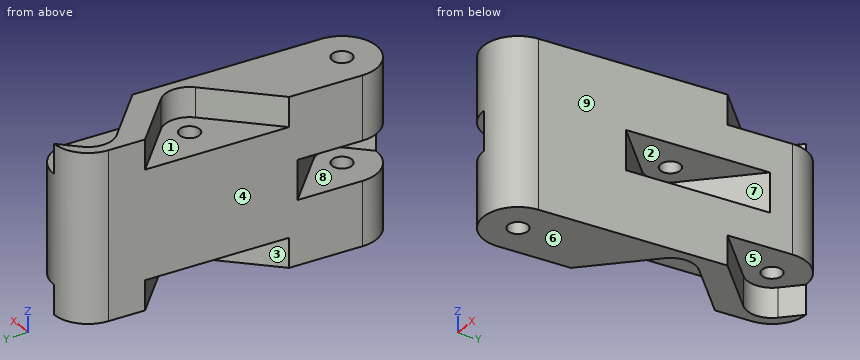
from build123d import *

# Parameters (mm, degrees)
SKETCH1_R           = 1
BOSS_EXTRUDE1_DEPTH = 8.5
CUT_EXTRUDE1_DEPTH  = 2
CUT_EXTRUDE2_START  = -3
CUT_EXTRUDE2_DEPTH  = 3


with BuildPart() as part:
    # Sketch1 → Boss-Extrude1 (new body)
    with BuildSketch(Plane.XY):
        with BuildLine():
            Line((12.42679356, 42.170979879), (10.789298219, 17.224665341))
            ThreePointArc((10.789298219, 17.224665341), (7.067564836, 13.961430653), (3.804330148, 17.683164036))
            Line((3.804330148, 17.683164036), (5.441825489, 42.629478574))
            ThreePointArc((5.441825489, 42.629478574), (9.163558872, 45.892713262), (12.42679356, 42.170979879))
        make_face()
        with Locations((7.296814184, 17.453914689)):
            Circle(SKETCH1_R, mode=Mode.SUBTRACT)
        with Locations((8.279311388, 32.421703411)):
            Circle(SKETCH1_R, mode=Mode.SUBTRACT)
        with Locations((8.934309525, 42.400229226)):
            Circle(SKETCH1_R, mode=Mode.SUBTRACT)
    boss_extrude1 = extrude(amount=BOSS_EXTRUDE1_DEPTH)

    # Sketch2 → Cut-Extrude1 (cut)
    # profile 1 of 2: a face of its own
    with BuildSketch(Plane(origin=(0, 0, 0), x_dir=(-1, 0, 0), z_dir=(0, 0, -1))):
        with BuildLine():
            ThreePointArc((-6.511544435, 30.653936458), (-5.779311388, 32.421703411), (-6.511544435, 34.189470364))
            Line((-6.511544435, 34.189470364), (-12.281634265, 39.959560194))
            Line((-12.281634265, 39.959560194), (-11.353008502, 25.812472391))
            Line((-11.353008502, 25.812472391), (-6.511544435, 30.653936458))
        make_face()
        with BuildLine():
            ThreePointArc((-7.279311388, 32.421703411), (-7.355431856, 32.039019979), (-7.572204607, 31.71459663))
            ThreePointArc((-7.572204607, 31.71459663), (-9.203190921, 32.804386844), (-7.279311388, 32.421703411))
        make_face(mode=Mode.SUBTRACT)
    # profile 2 of 2: a face of its own
    with BuildSketch(Plane(origin=(0, 0, 0), x_dir=(-1, 0, 0), z_dir=(0, 0, -1))):
        with BuildLine():
            ThreePointArc((-9.064581137, 19.221681642), (-9.796814184, 17.453914689), (-9.064581137, 15.686147736))
            Line((-9.064581137, 15.686147736), (-3.30921397, 9.930780569))
            Line((-3.30921397, 9.930780569), (-3.30921397, 24.977048808))
            Line((-3.30921397, 24.977048808), (-9.064581137, 19.221681642))
        make_face()
    cut_extrude1 = extrude(amount=-CUT_EXTRUDE1_DEPTH, mode=Mode.SUBTRACT)

    # Sketch3 → Cut-Extrude2 (cut)
    with BuildSketch(Plane.XY.offset(8.5).offset(CUT_EXTRUDE2_START)):
        with BuildLine():
            Line((7.166542572, 44.167996179), (14.185239134, 51.186692741))
            Line((14.185239134, 51.186692741), (14.789130122, 33.009874723))
            Line((14.789130122, 33.009874723), (7.166542572, 40.632462273))
            ThreePointArc((7.166542572, 40.632462273), (6.434309525, 42.400229226), (7.166542572, 44.167996179))
        make_face()
        with BuildLine():
            Line((10.047078341, 34.189470364), (4.005126991, 40.231421715))
            Line((4.005126991, 40.231421715), (3.260559385, 23.867417502))
            Line((3.260559385, 23.867417502), (10.047078341, 30.653936458))
            ThreePointArc((10.047078341, 30.653936458), (10.779311388, 32.421703411), (10.047078341, 34.189470364))
        make_face()
    cut_extrude2 = extrude(amount=CUT_EXTRUDE2_DEPTH, mode=Mode.SUBTRACT)

    # Mirror1: Boss-Extrude1, Cut-Extrude1, Cut-Extrude2 across plane
    add(boss_extrude1.mirror(Plane(origin=(0, 0, 0), x_dir=(1, 0, 0), z_dir=(0, 0, -1))))
    add(cut_extrude1.mirror(Plane(origin=(0, 0, 0), x_dir=(1, 0, 0), z_dir=(0, 0, -1))), mode=Mode.SUBTRACT)
    add(cut_extrude2.mirror(Plane(origin=(0, 0, 0), x_dir=(1, 0, 0), z_dir=(0, 0, -1))), mode=Mode.SUBTRACT)


solid = part.part
Source: CAD feature listing. Evaluate the final solid. Frame: model axes, mm. Face numbers are marked on the shaded views. A direction names the side the tool comes from. Give positions to 0.01 mm unless a question says otherwise; leave off trailing zeros. Write each loop counter-clockwise with the first axis right and the second up, starting at its lowest first coordinate (ties: lowest second). Pieces come first, ordered by that corner, then holes. Notation, with made-up numbers: M 25,46 L 72,46 A15 ccw 72,66 Z; hole C 80,36.25 d10. An arc over 180 degrees is marked long. Answer as a JSON object with one key per item and string values.
Q1. Access query for the marked faces 1, 2, 3, 4 and 5. Directions: +Z, -Z, +X, -X, +Y, -Y. A direction counts if a zero-diameter tool reaches every point of the face in a straight line with its end or side. Return the directions, or none.
Geometry check:
{"face 1": "+Z, -X", "face 2": "+X", "face 3": "-Z, -X", "face 4": "+Z, -Z, -X, +Y", "face 5": "-Z, +X"}
Q2. Cut plane B-B, the plane y = 18. Return the cut outline in (x, z).
Geometry check:
{"outline": "M 3.83,-8.5 L 6.46,-8.5 L 6.46,-2 L 3.83,-2 Z; M 3.83,2 L 6.46,2 L 6.46,8.5 L 3.83,8.5 Z; M 8.13,-8.5 L 10.84,-8.5 L 10.84,8.5 L 8.13,8.5 L 8.13,2 L 9.74,2 L 9.74,-2 L 8.13,-2 Z"}
Q3. Mould query, pull axis Y, two halves, no side actions, for the marked faces 6, 7, 8 and 9. Classes: +Y half, -Y half, draft (parallel to the pull), parting line (faces both ways), or undercut.
Geometry check:
{"face 6": "draft", "face 7": "undercut", "face 8": "undercut", "face 9": "-Y half"}
Q4. Cut plane C-C, the plane y = 39.5. Return the cut outline in (x, z), then the cut area to 3 significant figures.
Geometry check:
{"outline": "M 5.24,-8.5 L 8.3,-8.5 L 8.3,-5.5 L 12.25,-5.5 L 12.25,-2 L 11.82,-2 L 11.82,2 L 12.25,2 L 12.25,5.5 L 8.3,5.5 L 8.3,8.5 L 5.24,8.5 Z", "area": "93.8 mm^2"}
Q5. Contact query for flat-ended pins moving along their axis: P1, Ø1.5, axis at y = 21.5, z = 2, coming from the -X side; P2, Ø5, axis at y = 29.5, z = -0.5, coming from the -X side; P3, Ø2.5, axis at x = 8.93, y = 42.4, coming from the -Z side. Output: stop coordinate, or through.
Geometry check:
{"P1": "stops at x = 4.01", "P2": "stops at x = 4.42", "P3": "stops at z = -5.5"}
Q6. Ray query, line 1 along Z through (x, y) = (9.5, 37); line 2 along Y through (x, z) = (7.5, -4); line 3 along Y through (x, z) = (6, 0.75). Return the intervals inside material, ascending.
Geometry check:
{"line 1": "z = -8.5 to -2, 2 to 8.5", "line 2": "y = 13.96 to 16.47, 18.43 to 31.8, 33.05 to 45.59", "line 3": "y = 22.29 to 31.39, 33.45 to 44.31"}
Q7. Cut plane D-D, the plane z = -1.25. Return the cut outline in (x, y), then the cut area to 3 significant figures.
Geometry check:
{"outline": "M 4.22,24.06 L 9.06,19.22 A2.5 cw 9.06,15.69 L 7.33,13.95 A3.5 ccw 10.79,17.22 L 11.35,25.81 L 6.51,30.65 A2.5 cw 6.51,34.19 L 12.28,39.96 L 12.43,42.17 A3.5 ccw 5.44,42.63 Z; hole C 8.93,42.4 d2", "area": "124 mm^2"}
Q8. Cut plane A-A, the plane z = 2.5. Return the cut outline in (x, y).
Geometry check:
{"outline": "M 3.8,17.68 A3.5 ccw 10.79,17.22 L 12.43,42.17 A3.5 ccw 5.44,42.63 Z; hole C 7.3,17.45 d2; hole C 8.28,32.42 d2; hole C 8.93,42.4 d2"}
